```python
from build123d import *

# Parameters (mm, degrees)
SKETCH1_W                                      = 25.4
SKETCH1_H                                      = 38.1
SKETCH1_W_2                                    = 50.8
BOSS_EXTRUDE1_DEPTH                            = 6.35
SKETCH1_3_W                                    = 50.8
SKETCH1_3_H                                    = 38.1
SKETCH1_3_W_2                                  = 25.4
BOSS_EXTRUDE2_DEPTH                            = 6.35
CBORE_FOR_8_SOCKET_HEAD_CAP_SCREW1_D           = 4.4958
CBORE_FOR_8_SOCKET_HEAD_CAP_SCREW1_DEPTH       = 6.35
CBORE_FOR_8_SOCKET_HEAD_CAP_SCREW1_CBORE_D     = 7.9375
CBORE_FOR_8_SOCKET_HEAD_CAP_SCREW1_CBORE_DEPTH = 4.1656
F_8_32_TAPPED_HOLE1_D                          = 3.4544


with BuildPart() as part:
    # Sketch1 → Boss-Extrude1 (new body)
    with BuildSketch(Plane(origin=(0, 0, 0), x_dir=(1, 0, 0), z_dir=(0, 1, 0))):
        with Locations((-38.1, 0)):
            Rectangle(SKETCH1_W, SKETCH1_H)
        Rectangle(SKETCH1_W_2, SKETCH1_H)
    extrude(amount=-BOSS_EXTRUDE1_DEPTH)

    # Sketch1<3> → Boss-Extrude2 (add)
    with BuildSketch(Plane(origin=(0, 0, 0), x_dir=(1, 0, 0), z_dir=(0, 1, 0))):
        Rectangle(SKETCH1_3_W, SKETCH1_3_H)
        with Locations((38.1, 0)):
            Rectangle(SKETCH1_3_W_2, SKETCH1_3_H)
    extrude(amount=BOSS_EXTRUDE2_DEPTH)

    # CBORE for #8 Socket Head Cap Screw1
    with Locations(Plane(origin=(0, -6.35, 0), x_dir=(-1, 0, 0), z_dir=(0, -1, 0))):
        with Locations((31.75, 10.998522628), (44.45, -10.998522628)):
            CounterBoreHole(CBORE_FOR_8_SOCKET_HEAD_CAP_SCREW1_D / 2, CBORE_FOR_8_SOCKET_HEAD_CAP_SCREW1_CBORE_D / 2, CBORE_FOR_8_SOCKET_HEAD_CAP_SCREW1_CBORE_DEPTH, depth=CBORE_FOR_8_SOCKET_HEAD_CAP_SCREW1_DEPTH)

    # #8-32 Tapped Hole1 (through all)
    with Locations(Plane(origin=(0, 0, 0), x_dir=(-1, 0, 0), z_dir=(0, -1, 0))):
        with Locations((-31.75, 10.998522628), (-44.45, -10.998522628)):
            Hole(F_8_32_TAPPED_HOLE1_D / 2)


solid = part.part
```
Work out the finished part from the listing and answer in its coordinate system (mm). A direction names the side the tool comes from. Round coordinates to 2 decimals unless told otherwise and drop trailing zeros. Write each loop counter-clockwise with the first axis right and the second up, starting at its lowest first coordinate (ties: lowest second). Pieces come first, ordered by that corner, then holes. Notation, with made-up numbers: (3.25, 59) -> (52.25, 59) arc R10 cw to (52.25, 74) -> close; hole circle Ø10 at (23.5, 17). An arc over 180 degrees is marked (long way). Write each question's results on one line, items separated by ' | '.
Q1. Straight lines are drawn through the part: line 1 along Z through (x, y) = (-31.75, -0.5); line 2 along Z through (x, y) = (44.45, 1.75); line 3 along Y through (x, z) = (47.5, -12.5). For each, find the intervals that lie inside material, in ascending order. Write a range as [from, to].
Data:
line 1: [-19.05, -13.25], [-8.75, 19.05] | line 2: [-19.05, 9.27], [12.73, 19.05] | line 3: [0, 6.35]
Q2. Section D-D, the plane x = 44.45 is taken. Write down the section's boundary in (y, z), then the cut area to 3 significant figures.
Data:
outline: (0, -19.05) -> (6.35, -19.05) -> (6.35, 9.27) -> (0, 9.27) -> close; (0, 12.73) -> (6.35, 12.73) -> (6.35, 19.05) -> (0, 19.05) -> close | area: 220 mm^2
Q3. Determine the mould class of faces 1 (the flat face through (1, 0, -19.05)), 2 (the flat face through (-50.8, -3, 0)), 3 (the flat face through (-46, -2.184, 13)) for opening direction Z: released by +Z, released by -Z, zero draft, split by the parting line, or undercut.
Data:
face 1: released by -Z | face 2: zero draft | face 3: undercut
Q4. Flat-ended cylindrical pins translate along their axes: P1, Ø5, axis at y = 4.5, z = -4, coming from the -X side; P2, Ø1.9, axis at y = -3.5, z = 3.5, coming from the +X side; P3, Ø5, axis at x = -44.45, z = 11, coming from the -Y side; P4, Ø3, axis at x = 44.45, z = 11, coming from the -Y side. Find the tip coordinate at first contact, or state that the pin passes through.
Data:
P1: x = -25.4 | P2: x = 25.4 | P3: y = -2.18 | P4: through
Q5. Section B-B, the plane z = 6 is taken. Write down the section's boundary in (x, y), then the cut area to 3 significant figures.
Data:
outline: (-50.8, -6.35) -> (25.4, -6.35) -> (25.4, 0) -> (50.8, 0) -> (50.8, 6.35) -> (-25.4, 6.35) -> (-25.4, 0) -> (-50.8, 0) -> close | area: 968 mm^2
Q6. Section A-A, the plane x = -31.75 is taken. Write down the section's boundary in (y, z).
Data:
outline: (-6.35, -19.05) -> (0, -19.05) -> (0, -13.25) -> (-2.18, -13.25) -> (-2.18, -14.97) -> (-6.35, -14.97) -> close; (-6.35, -7.03) -> (-2.18, -7.03) -> (-2.18, -8.75) -> (0, -8.75) -> (0, 19.05) -> (-6.35, 19.05) -> close
Q7. Which of the six approach directions +Z, -Z, +X, -X, +Y, -Y give full straight-line access (tool end or side, diameter ignored) to faces 4 (the flat face through (-33.5, -2.184, -9.3)), 5 (the flat face through (25.4, -3, 0)), 6 (the flat face through (-25.4, 3, 0)), 7 (the flat face through (12, 6.35, 0))?
Data:
face 4: -Y | face 5: +Z, -Z, +X, -Y | face 6: +Z, -Z, -X, +Y | face 7: +Z, -Z, +X, -X, +Y
Q8. Section C-C, the plane y = 4.5 is taken. Write down the section's boundary in (x, z), then the cut area to 3 significant figures.
Data:
outline: (-25.4, -19.05) -> (50.8, -19.05) -> (50.8, 19.05) -> (-25.4, 19.05) -> close; hole circle Ø3.45 at (31.75, -11); hole circle Ø3.45 at (44.45, 11) | area: 2,880 mm^2
